Study the drawing (mm; zero at the part's minimum x, y, z) and answer. A direction names the side the tool comes from. Round coordinates to 2 decimals unless told otherwise and drop trailing zeros. Order: outer loops, then holes, each group sorted by start corner. A loop starts at its lowest first (then second) coordinate and runs counter-clockwise, first axis right, second up. Notation, with made-up numbers: (52, 89.5) -> (77, 89.5) arc R14 cw to (77, 107.5) -> close; hole circle Ø2 at (23, 34.5). An arc over 180 degrees is marked (long way). Answer in a Markdown table with one row per item. Add a question column.
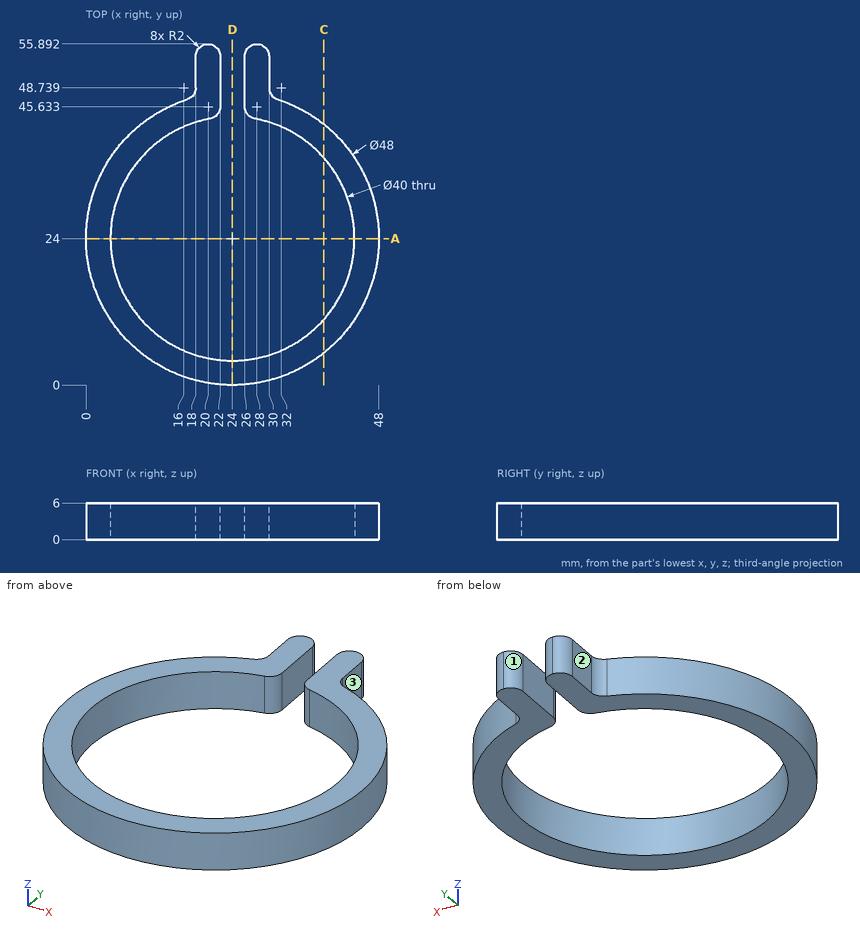
Item 1: The part is cut by section C-C, the plane x = 39. Give the vertices of the cut face in (y, z) (1 decimal).
Item 2: The part is cut by section D-D, the plane x = 24. Give the vertices of the cut face in (y, z), and give its area (3 significant figures).
Item 3: Find the intervals of material crossed by probe 1 along X at (y, z) = (24, 2.1); probe 2 along Y at (x, z) = (24, 2.1); probe 3 along Y at (x, z) = (28.5, 1.55) (1 decimal), in increasing order. Write a range as [from, to].
Item 4: A tool of negligible diameter and unlimited length cuts with its end or side. For the marked faces 1, 2 and 3, from which of +Z, -Z, +X, -X, +Y, -Y can it reach the whole face along a straight path? Write none if from no direction.
Item 5: The part is cut by section A-A, the plane y = 24. Give the vertices of the cut face in (x, z).
Item 6: Flat-ended cylindrical pins translate along their axes: P1, Ø2.5, axis at y = 50.5, z = 2.5, coming from the -X side; P2, Ø1.8, axis at y = 49, z = 1.5, coming from the +X side (1 decimal); P3, Ø4, axis at x = 5.5, y = 19, coming from the +Z side. Find the tip coordinate at first contact, or state that the pin passes through.
Resolved:
| question | item | result |
|---|---|---|
| 1 | outline | (5.3, 0) -> (10.8, 0) -> (10.8, 6) -> (5.3, 6) -> close; (37.2, 0) -> (42.7, 0) -> (42.7, 6) -> (37.2, 6) -> close |
| 2 | outline | (0, 0) -> (4, 0) -> (4, 6) -> (0, 6) -> close |
| 2 | area | 24.0 mm2 |
| 3 | probe 1 | [0, 4], [44, 48] |
| 3 | probe 2 | [0, 4] |
| 3 | probe 3 | [0.4, 4.5], [43.5, 55.8] |
| 4 | face 1 | +Z, -Z, +Y |
| 4 | face 2 | +Z, -Z, -X, +Y |
| 4 | face 3 | +Z, -Z, +X, +Y |
| 5 | outline | (0, 0) -> (4, 0) -> (4, 6) -> (0, 6) -> close; (44, 0) -> (48, 0) -> (48, 6) -> (44, 6) -> close |
| 6 | P1 | x = 18 |
| 6 | P2 | x = 30.1 |
| 6 | P3 | z = 6 |
